Source: three-view drawing plus pictorial views. Frame: mm from the lowest corner of the part. A direction names the side the tool comes from. Coordinates: 2 decimals unless noted, no trailing zeros. Write each loop counter-clockwise with the first axis right and the second up, starting at its lowest first coordinate (ties: lowest second). Pieces come first, ordered by that corner, then holes. Notation, with made-up numbers: (73.5, -3) -> (126.5, -3) arc R24 ccw to (126.5, 15) -> close; hole circle Ø7 at (67.25, 69). An arc over 180 degrees is marked (long way). One line per item, written item: value.
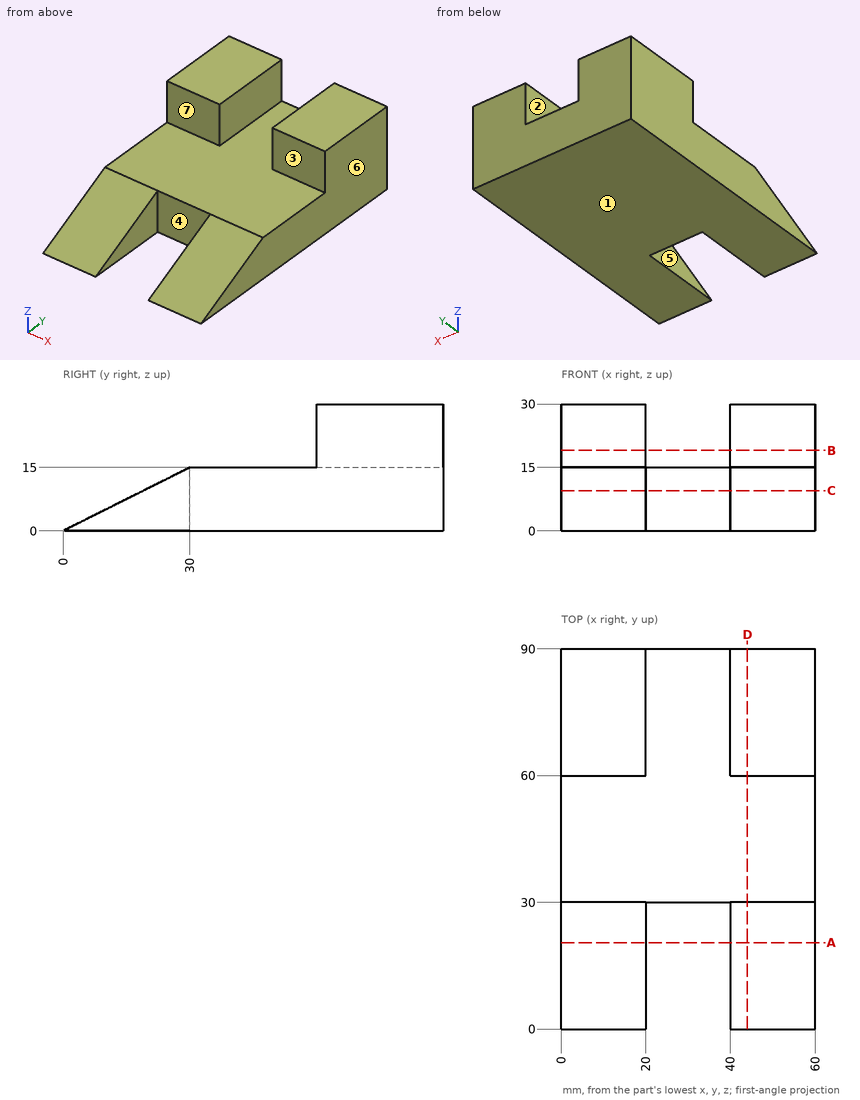
(1) Section C-C (z = 9.5). Return the cut outline in (x, y).
Responses:
outline: (0, 19) -> (20, 19) -> (20, 30) -> (40, 30) -> (40, 19) -> (60, 19) -> (60, 90) -> (0, 90) -> close
(2) Section A-A (y = 20.5). Return the cut outline in (x, z), then the cut area to 3 significant figures.
Responses:
outline: (0, 0) -> (20, 0) -> (20, 10.25) -> (0, 10.25) -> close; (40, 0) -> (60, 0) -> (60, 10.25) -> (40, 10.25) -> close
area: 410 mm2
(3) Line query: line 1 (X direction, y = 27, z = 6); line 2 (Z direction, x = 12, y = 59); line 3 (Y direction, x = 28.5, z = 11.5). Output: solid intervals per line, ascending. Write a range as [from, to].
Responses:
line 1: x = [0, 20], [40, 60]
line 2: z = [0, 15]
line 3: y = [30, 90]
(4) Section D-D (x = 44). Return the cut outline in (y, z).
Responses:
outline: (0, 0) -> (90, 0) -> (90, 30) -> (60, 30) -> (60, 15) -> (30, 15) -> close
(5) First-contact query: pin 1 (12 mm diameter, centred on x = 9, z = 25, fed in from -Y); pin 2 (16.5 mm diameter, centred on y = 10.5, z = 7.5, fed in from -X); pin 3 (1.5 mm diameter, centred on x = 23, z = 13, fed in from -Y); pin 4 (1 mm diameter, centred on x = 8, z = 6.5, fed in from -Y). Flat tips, straight axial feed; report the tip coordinate or a pass-through.
Responses:
pin 1: stops at y = 60
pin 2: stops at x = 0
pin 3: stops at y = 30
pin 4: stops at y = 12
(6) Section B-B (z = 19). Return the cut outline in (x, y), then the cut area to 3 significant figures.
Responses:
outline: (0, 60) -> (20, 60) -> (20, 90) -> (0, 90) -> close; (40, 60) -> (60, 60) -> (60, 90) -> (40, 90) -> close
area: 1,200 mm2
(7) Reachability of the marked faces 1, 2, 3 and 4 from +Z, -Z, +X, -X, +Y, -Y: full face, straight path, thin tool, end or side. Return the list, or none.
Responses:
face 1: -Z, +X, -X, +Y, -Y
face 2: +Z, +Y, -Y
face 3: +Z, +X, -X, -Y
face 4: +Z, -Z, -Y
(8) Pull-direction query (X, two-part tool) for the marked faces 5, 6 and 7; classes: released by +X, released by -X, zero draft, split by the parting line, or undercut.
Responses:
face 5: undercut
face 6: released by +X
face 7: zero draft
